Input: part model. Units: mm. Frame: model coordinates. A direction names the side the tool comes from. Round coordinates to 2 decimals unless told otherwise and drop trailing zeros. Write each loop counter-clockwise with the first axis right and the second up, starting at its lowest first coordinate (ties: lowest second). Pieces come first, ordered by that corner, then holes. Notation, with made-up numbers: (-32, 42) -> (-4, 42) arc R19 ccw to (-4, 76) -> close; hole circle Ø11 at (-8.75, 27.5). An arc over 180 degrees is marked (long way). Write item = value, one per line. Start each with the question number.
```python
from build123d import *

# Parameters (mm, degrees)
F2_R     = 3.25
F2_R_2   = 1.75
F3_DEPTH = 4
F4_DEPTH = 4.001
F5_DEPTH = 2
F6_SIZE  = 2


with BuildPart() as f3:
    # F2 (on Top) → F3 (new body)
    with BuildSketch(Plane.XY):
        Polygon((0, 60), (0, 0), (60, 0), (60, 20), (20, 20), (20, 60), align=None)
        with Locations((10, 10)):
            Circle(F2_R, mode=Mode.SUBTRACT)
        with Locations((30, 10)):
            Circle(F2_R, mode=Mode.SUBTRACT)
        with Locations((50, 10)):
            Circle(F2_R, mode=Mode.SUBTRACT)
        with Locations((10, 30)):
            Circle(F2_R, mode=Mode.SUBTRACT)
        with Locations((10, 50)):
            Circle(F2_R, mode=Mode.SUBTRACT)
        with Locations((10, 50)):
            Circle(F2_R)
        with Locations((10, 50)):
            Circle(F2_R_2, mode=Mode.SUBTRACT)
        with Locations((10, 30)):
            Circle(F2_R)
        with Locations((10, 30)):
            Circle(F2_R_2, mode=Mode.SUBTRACT)
        with Locations((10, 10)):
            Circle(F2_R)
        with Locations((10, 10)):
            Circle(F2_R_2, mode=Mode.SUBTRACT)
        with Locations((30, 10)):
            Circle(F2_R)
        with Locations((30, 10)):
            Circle(F2_R_2, mode=Mode.SUBTRACT)
        with Locations((50, 10)):
            Circle(F2_R)
        with Locations((50, 10)):
            Circle(F2_R_2, mode=Mode.SUBTRACT)
        with Locations((10, 50)):
            Circle(F2_R_2)
        with Locations((10, 30)):
            Circle(F2_R_2)
        with Locations((10, 10)):
            Circle(F2_R_2)
        with Locations((30, 10)):
            Circle(F2_R_2)
        with Locations((50, 10)):
            Circle(F2_R_2)
    extrude(amount=-F3_DEPTH)

    # F2 (on Top) → F4 (cut, through all)
    with BuildSketch(Plane.XY):
        with Locations((10, 50)):
            Circle(F2_R_2)
        with Locations((10, 30)):
            Circle(F2_R_2)
        with Locations((10, 10)):
            Circle(F2_R_2)
        with Locations((30, 10)):
            Circle(F2_R_2)
        with Locations((50, 10)):
            Circle(F2_R_2)
    extrude(amount=-F4_DEPTH, mode=Mode.SUBTRACT)

    # F2 (on Top) → F5 (cut)
    with BuildSketch(Plane.XY):
        with Locations((10, 50)):
            Circle(F2_R)
        with Locations((10, 50)):
            Circle(F2_R_2, mode=Mode.SUBTRACT)
        with Locations((10, 30)):
            Circle(F2_R)
        with Locations((10, 30)):
            Circle(F2_R_2, mode=Mode.SUBTRACT)
        with Locations((10, 10)):
            Circle(F2_R)
        with Locations((10, 10)):
            Circle(F2_R_2, mode=Mode.SUBTRACT)
        with Locations((30, 10)):
            Circle(F2_R)
        with Locations((30, 10)):
            Circle(F2_R_2, mode=Mode.SUBTRACT)
        with Locations((50, 10)):
            Circle(F2_R)
        with Locations((50, 10)):
            Circle(F2_R_2, mode=Mode.SUBTRACT)
    extrude(amount=-F5_DEPTH, mode=Mode.SUBTRACT)

    # F6
    f6_edges = [f3.edges().sort_by_distance(p)[0] for p in [
        (40, 20, 0),
        (20, 40, 0),
        (10, 60, 0),
        (0, 30, 0),
        (30, 0, 0),
        (60, 10, 0),
    ]]
    chamfer(f6_edges, length=F6_SIZE)


solid = f3.part
```
1. Section C-C (z = -3.1). Output: boundary loops of the cut face in (x, y).
2. Pin query (flat end, axial travel): P1, Ø1, axis at y = 43, z = -3, coming from the +X side; P2, Ø3, axis at x = 50, y = 10, coming from the +Z side; P3, Ø1, axis at x = 19.5, y = 51.5, coming from the +Z side; P4, Ø4, axis at x = 30, y = 10, coming from the +Z side. Return the tip coordinate at first contact, or that it passes through.
3. Reachability of faces 4 (the cylindrical face through (33.1, 10.98, -0.99)), 5 (the flat face through (39, 19, -1)), 6 (the flat face through (20, 40, -3)), 7 (the flat face through (60, 10, -3)), 8 (the cylindrical face through (28.25, 10.08, -2.99)) from +Z, -Z, +X, -X, +Y, -Y: full face, straight path, thin tool, end or side. Return the list, or none.
4. Line query: line 1 along Y through (x, z) = (10, -2.75); line 2 along Y through (x, z) = (7.5, -1.9); line 3 along X through (y, z) = (45.5, -2.3). Output: solid intervals per line, ascending.
5. Section A-A (x = 10). State how many separate pieces and enclosed holes the cut face has, then the cut area to 3 significant figures.
6. Mould query, pull axis X, two halves, no side actions, for faces 1 (the flat face through (11.4, 48.6, -2)), 2 (the flat face through (17, 24, 0)), 3 (the flat face through (59, 10, -1)). Classes: pulls with the +X half, pulls with the -X half, needs draft (parallel to the pull), parting line crosses it, or undercut.
7. Section D-D (x = 30). Output: boundary loops of the cut face in (y, z).
Check sheet entries:
q1.outline = (0, 0) -> (60, 0) -> (60, 20) -> (20, 20) -> (20, 60) -> (0, 60) -> close; hole circle Ø3.5 at (10, 10); hole circle Ø3.5 at (10, 30); hole circle Ø3.5 at (10, 50); hole circle Ø3.5 at (30, 10); hole circle Ø3.5 at (50, 10)
q2.P1 = 20
q2.P2 = through
q2.P3 = -1
q2.P4 = -2
q3.face_4 = +Z
q3.face_5 = +Z, +X, +Y
q3.face_6 = +Z, -Z, +X, +Y
q3.face_7 = +Z, -Z, +X, +Y, -Y
q3.face_8 = +Z, -Z
q4.line_1 = 0 to 8.25, 11.75 to 28.25, 31.75 to 48.25, 51.75 to 60
q4.line_2 = 0.1 to 7.92, 12.08 to 27.92, 32.08 to 47.92, 52.08 to 59.9
q4.line_3 = 0 to 20
q5.separate_pieces = 4
q5.enclosed_holes = 0
q5.area = 176 mm2
q6.face_1 = undercut
q6.face_2 = needs draft
q6.face_3 = pulls with the +X half
q7.outline = (0, -4) -> (8.25, -4) -> (8.25, -2) -> (6.75, -2) -> (6.75, 0) -> (2, 0) -> (0, -2) -> close; (11.75, -4) -> (20, -4) -> (20, -2) -> (18, 0) -> (13.25, 0) -> (13.25, -2) -> (11.75, -2) -> close
